from build123d import *

# Parameters (mm, degrees)
SKETCH2_R           = 145
SKETCH2_R_2         = 105
BOSS_EXTRUDE1_START = -50
SKETCH6_R           = 15
SKETCH6_R_2         = 145
BOSS_EXTRUDE1_DEPTH = 50
CHAMFER1_SIZE       = 10
FILLET1_R           = 10
SKETCH7_R           = 15
SKETCH7_R_2         = 145
BOSS_EXTRUDE2_DEPTH = 50
CHAMFER2_SIZE       = 10
FILLET2_R           = 10
SKETCH9_R           = 30
CUT_EXTRUDE1_DEPTH  = 10
SKETCH10_R          = 30
CUT_EXTRUDE2_DEPTH  = 10


with BuildPart() as part:
    # Sweep1: sweep along a path in Sketch1
    with BuildLine(Plane.XY) as sweep1_path:
        Line((0, 0), (-150, 0))
        ThreePointArc((-150, 0), (-333.847763109, 76.152236891), (-410, 260))
        Line((-410, 260), (-410, 410))
    # Sketch2 → Sweep1 (sweep)
    with BuildSketch(Plane(origin=(-410, 410, 0), x_dir=(1, 0, 0), z_dir=(0, 1, 0))):
        Circle(SKETCH2_R)
        Circle(SKETCH2_R_2, mode=Mode.SUBTRACT)
    sweep(path=sweep1_path.line)

    # Sketch6 → Boss-Extrude1 (add)
    with BuildSketch(Plane(origin=(0, 0, 0), x_dir=(0, 0, -1), z_dir=(1, 0, 0)).offset(BOSS_EXTRUDE1_START)):
        with BuildLine():
            Line((-160, -180), (160, -180))
            ThreePointArc((160, -180), (174.142135624, -174.142135624), (180, -160))
            Line((180, -160), (180, 160))
            ThreePointArc((180, 160), (174.142135624, 174.142135624), (160, 180))
            Line((160, 180), (-160, 180))
            ThreePointArc((-160, 180), (-174.142135624, 174.142135624), (-180, 160))
            Line((-180, 160), (-180, -160))
            ThreePointArc((-180, -160), (-174.142135624, -174.142135624), (-160, -180))
        make_face()
        with Locations((130, 130)):
            Circle(SKETCH6_R, mode=Mode.SUBTRACT)
        with Locations((130, -130)):
            Circle(SKETCH6_R, mode=Mode.SUBTRACT)
        with Locations((-130, -130)):
            Circle(SKETCH6_R, mode=Mode.SUBTRACT)
        with Locations((-130, 130)):
            Circle(SKETCH6_R, mode=Mode.SUBTRACT)
        with Locations(Location((0, 0, 0), (0, 0, 270))):
            Circle(SKETCH6_R_2, mode=Mode.SUBTRACT)
    extrude(amount=BOSS_EXTRUDE1_DEPTH)

    # Chamfer1
    chamfer1_edges = [part.edges().sort_by_distance(p)[0] for p in [
        (0, -105, 0),
    ]]
    chamfer(chamfer1_edges, length=CHAMFER1_SIZE)

    # Fillet1
    fillet1_edges = [part.edges().sort_by_distance(p)[0] for p in [
        (-50, -145, 0),
    ]]
    fillet(fillet1_edges, radius=FILLET1_R)

    # Sketch7 → Boss-Extrude2 (add)
    with BuildSketch(Plane(origin=(0, 410, 0), x_dir=(1, 0, 0), z_dir=(0, 1, 0))):
        with BuildLine():
            Line((-570, -180), (-250, -180))
            ThreePointArc((-250, -180), (-235.857864376, -174.142135624), (-230, -160))
            Line((-230, -160), (-230, 160))
            ThreePointArc((-230, 160), (-235.857864376, 174.142135624), (-250, 180))
            Line((-250, 180), (-570, 180))
            ThreePointArc((-570, 180), (-584.142135624, 174.142135624), (-590, 160))
            Line((-590, 160), (-590, -160))
            ThreePointArc((-590, -160), (-584.142135624, -174.142135624), (-570, -180))
        make_face()
        with Locations(Location((-540, 130, 0), (0, 0, 180))):
            Circle(SKETCH7_R, mode=Mode.SUBTRACT)
        with Locations(Location((-540, -130, 0), (0, 0, 180))):
            Circle(SKETCH7_R, mode=Mode.SUBTRACT)
        with Locations(Location((-280, -130, 0), (0, 0, 180))):
            Circle(SKETCH7_R, mode=Mode.SUBTRACT)
        with Locations(Location((-280, 130, 0), (0, 0, 180))):
            Circle(SKETCH7_R, mode=Mode.SUBTRACT)
        with Locations(Location((-410, 0, 0), (0, 0, 180))):
            Circle(SKETCH7_R_2, mode=Mode.SUBTRACT)
    extrude(amount=-BOSS_EXTRUDE2_DEPTH)

    # Chamfer2
    chamfer2_edges = [part.edges().sort_by_distance(p)[0] for p in [
        (-515, 410, 0),
    ]]
    chamfer(chamfer2_edges, length=CHAMFER2_SIZE)

    # Fillet2
    fillet2_edges = [part.edges().sort_by_distance(p)[0] for p in [
        (-555, 360, 0),
    ]]
    fillet(fillet2_edges, radius=FILLET2_R)

    # Sketch9 → Cut-Extrude1 (cut)
    with BuildSketch(Plane(origin=(0, 410, 0), x_dir=(1, 0, 0), z_dir=(0, 1, 0))):
        with Locations(Location((-540, 130, 0), (0, 0, 180))):
            Circle(SKETCH9_R)
        with Locations(Location((-280, 130, 0), (0, 0, 180))):
            Circle(SKETCH9_R)
        with Locations(Location((-540, -130, 0), (0, 0, 180))):
            Circle(SKETCH9_R)
        with Locations(Location((-280, -130, 0), (0, 0, 180))):
            Circle(SKETCH9_R)
    extrude(amount=-CUT_EXTRUDE1_DEPTH, mode=Mode.SUBTRACT)

    # Sketch10 → Cut-Extrude2 (cut)
    with BuildSketch(Plane(origin=(0, 0, 0), x_dir=(0, 0, -1), z_dir=(1, 0, 0))):
        with Locations((-130, 130)):
            Circle(SKETCH10_R)
        with Locations((130, 130)):
            Circle(SKETCH10_R)
        with Locations((-130, -130)):
            Circle(SKETCH10_R)
        with Locations((130, -130)):
            Circle(SKETCH10_R)
    extrude(amount=-CUT_EXTRUDE2_DEPTH, mode=Mode.SUBTRACT)


solid = part.part
Verification items for the finished model (mm, model axes). A direction names the side the tool comes from. Coordinates: 2 decimals unless noted, no trailing zeros. Order: outer loops, then holes, each group sorted by start corner. A loop starts at its lowest first (then second) coordinate and runs counter-clockwise, first axis right, second up. Notation, with made-up numbers: M -17,-1.75 L 41,-1.75 A23 ccw 41,12.25 Z; hole C -4,41 d10. An arc over 180 degrees is marked long. One line per item, written item: value. Start each with the question number.
Item 1: Sectioned sample at C-C (x = -280). Count the separate pieces of the cut face and the enclosed holes in it, then the cut area to 3 significant figures.
Item 2: Scan lines: probe 1 along Y at (x, z) = (-42, -130); probe 2 along X at (y, z) = (167, 19). Record each from-to range of solid material in increasing order.
Item 3: Gauge pin test, flat ends, axial feed: pin 1 (6 mm diameter, centred on x = -70, z = 104.5, fed in from -Y); pin 2 (8 mm diameter, centred on x = -157, z = 55, fed in from +Y); pin 3 (12 mm diameter, centred on y = 299.5, z = -64.5, fed in from -X). Record the tip position at first contact, or that the pin passes through.
Item 4: Access from +Z, -Z, +X, -X, +Y, -Y to the whole of each face (thin tool, end or side, straight path). Record for faces 1 (the flat face through (-412, 385, 180)), 2 (the flat face through (-413, 360, 157)), 3 (the cylindrical face through (-30.28, 140.138, 141.056)), 4 (the cylindrical face through (-293.843, 405.07, 103.385)), 5 (the flat face through (-230, 385, 2)).
Item 5: Sectioned sample at B-B (y = 293.5). Enter the section's corners in (x, z), then the cut area to 3 significant figures.
Item 6: Mould release check, pull along X, two halves, no side actions. Record for faces 6 (the flat face through (-266, 400, 124)), 7 (the cylindrical face through (-80.98, 100.15, -31.54)), 8 (the flat face through (-10, 144, -136)): released by +X, released by -X, zero draft, split by the parting line, or undercut.
Conclusion:
1. separate pieces: 3
1. enclosed holes: 1
1. area: 71,700 mm^2
2. probe 1: y = -180 to -145, -115 to 115, 145 to 180
2. probe 2: x = -542.89 to -501.16, -276.16 to -219.75, -50 to 0
3. pin 1: stops at y = -103.55
3. pin 2: stops at y = 135.95
3. pin 3: stops at x = -542.68
4. face 1: +Z, +X, -X, +Y, -Y
4. face 2: none
4. face 3: +X
4. face 4: +Y
4. face 5: +Z, -Z, +X, +Y
5. outline: C -410,0 d290; hole C -410,0 d210
5. area: 31,400 mm^2
6. face 6: undercut
6. face 7: zero draft
6. face 8: released by +X
